Design review of the part built by this model. Coordinates are the model's own, in mm. A direction names the side the tool comes from. Coordinates: 2 decimals unless noted, no trailing zeros. Write each loop counter-clockwise with the first axis right and the second up, starting at its lowest first coordinate (ties: lowest second). Pieces come first, ordered by that corner, then holes. Notation, with made-up numbers: (21.5, -0.5) -> (73.5, -0.5) arc R35 ccw to (73.5, 34.5) -> close; hole circle Ø8 at (68, 53.25). An arc over 180 degrees is marked (long way). Answer in a Markdown table with one row per item. Add a question column.
Item 1: Clearance check with flat-ended pins moving along their axes: P1, Ø6, axis at x = 28.5, z = -1, coming from the -Y side; P2, Ø1.5, axis at y = 96.5, z = -2.5, coming from the -X side; P3, Ø10, axis at y = 46.5, z = 4.5, coming from the +X side. State where each tip first meets the part, or that it passes through.
Item 2: Take a section at B-B, the plane z = 0. Write out the cut boundary in (x, y), and give its area (3 significant figures).
Item 3: Take a section at A-A, the plane x = 2. Write out the cut boundary in (y, z).
Item 4: Take a section at D-D, the plane z = 20. Write out the cut boundary in (x, y).
Item 5: To check wall thickness, follow line 1 (X direction, y = 90.5, z = 14.5); line 2 (X direction, y = 36.5, z = -9); line 3 (X direction, y = 24.5, z = 18). State the ranges of each line that lie inside material, in increasing order.
Item 6: Draft analysis for pull direction Y (two halves, no side actions). For faces 5 (the face through (-0.504, 26.094, 10.153)), 6 (the face through (-36, 17, 0)), 7 (the face through (22.488, 50.53, 21.855)), 8 (the face through (29, 3.5, 0)), state which applies: released by +Y, released by -Y, zero draft, split by the parting line, or undercut.
Item 7: For faces 1 (the face through (-24, 96, 0)), 2 (the face through (-9, 54, 3.75)), 3 (the face through (-0.34, 111.26, -4.81)), 4 (the face through (24, 96, 0)), list the 3-axis set-ups (+Z, -Z, +X, -X, +Y, -Y) from which the entire face can be reached by the end or side of a thin tool; tool diameter is ignored.
Item 8: Take a section at C-C, the plane y = 51.5. Write out the cut boundary in (x, z), and give its area (3 significant figures).
Autodesk Inventor part; units mm, degrees
ref_plane "Piano di lavoro2" through (0, 98, 15.8745) normal (0, 0.125, 0.9921567) x (-1, 0, 0)
ref_plane "YZ Plane" through (0, 0, 0) normal (1, 0, 0) x (0, 1, 0)
ref_plane "XZ Plane" through (0, 0, 0) normal (0, 1, 0) x (-1, 0, 0)
sketch "Schizzo1" plane through (0, 0, 0) normal (1, 0, 0) x (0, 1, 0)
  circle A0 centre (96, 0) radius 10
  circle A1 centre (96, 0) radius 16
  arc A2 (0, -15) -> (0, 15) centre (0, 0) ccw
  arc A3 (0, -28) -> (0, 28) centre (0, 0) ccw
  line L0 (0, 28) -> (0, 15)
  line L1 (0, -15) -> (0, -28)
  line L2 (0, -8.9606) -> (0, 0)
  line L3 (0, 0) -> (192, 0)
  line L4 (3.5, 27.7804) -> (98, 15.8745)
  line L5 (98, -15.8745) -> (3.5, -27.7804)
  line L6 (0, 15) -> (0, -15)
  point P0 (9.0471, 0)
  point P1 (0, -4.4803)
  dimension "d0" = 20
  dimension "d1" = 15
  dimension "d2" = 96
  dimension "d3" = 28
  dimension "d4" = 32
extrude "Estrusione1" add sketch "Schizzo1" along normal mid plane 48 contours L3 A0 | L3 A1 A0 | A0 L3 A1 | A0 L3
extrude "Estrusione2" add sketch "Schizzo1" along normal mid plane 72 contours L3 A2 L0 A3 | A3 L1 A2 L3
sketch "Schizzo3" plane through (0, 0, 0) normal (1, 0, 0) x (0, 1, 0)
  line L0 (98, 15.8745) -> (3.5, 27.7804)
  circle A0 centre (96, 0) radius 16
  arc A1 (0, -28) -> (0, 28) centre (0, 0) ccw
ref_plane "Piano di lavoro2" through (0, 98, 15.8745) normal (0, 0.125, 0.9921567) x (-1, 0, 0)
sketch "Schizzo4" plane through (0, 98, 15.8745) normal (0, 0.125, 0.9921567) x (-1, 0, 0)
  line L0 (24, -16) -> (24, 16)
  line L1 (-24, 16) -> (-24, -16)
  line L2 (36, 67.247) -> (36, 98.747)
  line L3 (-36, 98.747) -> (-36, 67.247)
  line L4 (0, 95.247) -> (0, 93.372) construction
  line L5 (-18, 0) -> (-33, 95.247)
  line L6 (-10.4076, 0) -> (-25.4076, 95.247)
  line L7 (18, 0) -> (33, 95.247)
  line L8 (10.4076, 0) -> (25.4076, 95.247)
  line L9 (0, 0) -> (0, 95.247)
  line L10 (18, 0) -> (10.4076, 0)
  line L11 (-10.4076, 0) -> (-18, 0)
  line L12 (-25.4076, 95.247) -> (-33, 95.247)
  line L13 (36, 93.372) -> (-36, 93.372)
  line L14 (33, 95.247) -> (25.4076, 95.247)
  line L15 (36, 97.122) -> (-36, 97.122)
  point P0 (36, 91.747)
  point P1 (-36, 91.747)
  dimension "d10" = 7.5
  dimension "d11" = 36
  dimension "d12" = 66
sketch "Schizzo6" plane through (0, 0, 0) normal (0, 0, 1) x (1, 0, 0)
  line L0 (-18, 98) -> (-33, 3.5)
  line L1 (-10.4076, 98) -> (-25.4076, 3.5)
  line L2 (10.4076, 98) -> (25.4076, 3.5)
  line L3 (18, 98) -> (33, 3.5)
  line L4 (-36, 0) -> (36, 0)
  line L5 (36, 0) -> (36, 0)
  line L6 (36, 0) -> (-36, 0)
  line L7 (-36, 0) -> (-36, 0)
  line L8 (-33, 3.5) -> (-25.4076, 3.5)
  line L9 (25.4076, 3.5) -> (33, 3.5)
  line L10 (-18, 98) -> (-10.4076, 98)
  line L11 (10.4076, 98) -> (18, 98)
  point P0 (0, 0)
extrude "Estrusione4" add sketch "Schizzo6" along normal up to surface surface through (0, 98, 15.8745) normal (0, 0.125, 0.9921567)
mirror "Specchio1" about plane through (0, 0, 0) normal (0, 0, 1) of "Estrusione4"
sketch "Schizzo8" plane through (0, 0, 0) normal (1, 0, 0) x (0, 1, 0)
  circle A0 centre (96, 0) radius 16
  arc A1 (0, -28) -> (0, 28) centre (0, 0) ccw
  line L0 (80.4457, 3.75) -> (27.7477, 3.75)
  line L1 (80.4457, -3.75) -> (27.7477, -3.75)
  line L2 (-22.7749, 0) -> (136.6494, 0) construction
  dimension "d17" = 7.5
extrude "Estrusione5" add sketch "Schizzo8" along normal up to surface contours A0 L1 A1 L0 surface through (10.4076, 98, 0) normal (-0.9876355, -0.1567675, 0)
extrude "Estrusione6" add sketch "Schizzo8" against normal up to surface contours A0 L1 A1 L0 surface through (-25.4076, 3.5, 0) normal (0.9876355, -0.1567675, 0)
sketch "Schizzo9" plane through (0, 0, 0) normal (0, 0, 1) x (1, 0, 0)
  line L0 (-50.4, 0) -> (50.4, 0)
  line L1 (0, -22.7749) -> (0, 136.6494)
  line L2 (-36, 28) -> (36, 28)
  line L3 (-13.194, 80.4457) -> (-21.5587, 27.7477)
  line L4 (21.5587, 27.7477) -> (13.194, 80.4457)
  line L5 (13.194, 80.4457) -> (-13.194, 80.4457)
  line L6 (-8.6349, 37) -> (8.6349, 37)
  line L7 (-10.6102, 39.3135) -> (-5.7776, 69.7592)
  line L8 (-3.8023, 71.4457) -> (3.8023, 71.4457)
  line L9 (5.7776, 69.7592) -> (10.6102, 39.3135)
  arc A0 (-3.8023, 71.4457) -> (-5.7776, 69.7592) centre (-3.8023, 69.4457) ccw
  arc A1 (5.7776, 69.7592) -> (3.8023, 71.4457) centre (3.8023, 69.4457) ccw
  arc A2 (-10.6102, 39.3135) -> (-8.6349, 37) centre (-8.6349, 39) ccw
  arc A3 (8.6349, 37) -> (10.6102, 39.3135) centre (8.6349, 39) ccw
  point P0 (0, 0)
  dimension "d22" = 9
  dimension "d23" = 9
  dimension "d24" = 2
extrude "Estrusione7" cut sketch "Schizzo9" along normal through all both and the other way through all contours L6 A2 L7 A0 L8 L1 | L1 L8 A1 L9 A3 L6
properties part number "05-15-2023 esercizi_piani parallaleli"
Answers:
| question | item | result |
|---|---|---|
| 1 | P1 | stops at y = 3.5 |
| 1 | P2 | stops at x = -24 |
| 1 | P3 | stops at x = 26.97 |
| 2 | outline | (-36, 15) -> (-31.17, 15) -> (-33, 3.5) -> (-25.41, 3.5) -> (-23.58, 15) -> (23.58, 15) -> (25.41, 3.5) -> (33, 3.5) -> (31.17, 15) -> (36, 15) -> (36, 28) -> (29.11, 28) -> (20.86, 80) -> (24, 80) -> (24, 112) -> (-24, 112) -> (-24, 80) -> (-20.86, 80) -> (-29.11, 28) -> (-36, 28) -> close; hole (-10.61, 39.31) arc R2 ccw to (-8.63, 37) -> (8.63, 37) arc R2 ccw to (10.61, 39.31) -> (5.78, 69.76) arc R2 ccw to (3.8, 71.45) -> (-3.8, 71.45) arc R2 ccw to (-5.78, 69.76) -> close |
| 2 | area | 4,680 mm^2 |
| 3 | outline | (0, -28) arc R28 ccw to (27.75, -3.75) -> (37, -3.75) -> (37, 3.75) -> (27.75, 3.75) arc R28 ccw to (0, 28) -> (0, 15) arc R15 cw to (0, -15) -> close; (71.45, -3.75) -> (80.45, -3.75) arc R16 ccw (long way) to (80.45, 3.75) -> (71.45, 3.75) -> close |
| 4 | outline | (-36, 0) -> (36, 0) -> (36, 19.6) -> (30.45, 19.6) -> (23.2, 65.25) -> (15.61, 65.25) -> (22.85, 19.6) -> (-22.85, 19.6) -> (-15.61, 65.25) -> (-23.2, 65.25) -> (-30.45, 19.6) -> (-36, 19.6) -> close |
| 5 | line 1 | x = -24 to 24 |
| 5 | line 2 | x = -27.76 to -20.17, 20.17 to 27.76 |
| 5 | line 3 | x = -29.67 to -22.07, 22.07 to 29.67 |
| 6 | face 5 | undercut |
| 6 | face 6 | zero draft |
| 6 | face 7 | released by +Y |
| 6 | face 8 | released by -Y |
| 7 | face 1 | +Z, -Z, -X, +Y |
| 7 | face 2 | +Z |
| 7 | face 3 | none |
| 7 | face 4 | +Z, -Z, +X, +Y |
| 8 | outline | (-25.38, -21.73) -> (-17.79, -21.73) -> (-17.79, -3.75) -> (-8.68, -3.75) -> (-8.68, 3.75) -> (-17.79, 3.75) -> (-17.79, 21.73) -> (-25.38, 21.73) -> close; (8.68, -3.75) -> (17.79, -3.75) -> (17.79, -21.73) -> (25.38, -21.73) -> (25.38, 21.73) -> (17.79, 21.73) -> (17.79, 3.75) -> (8.68, 3.75) -> close |
| 8 | area | 797 mm^2 |
